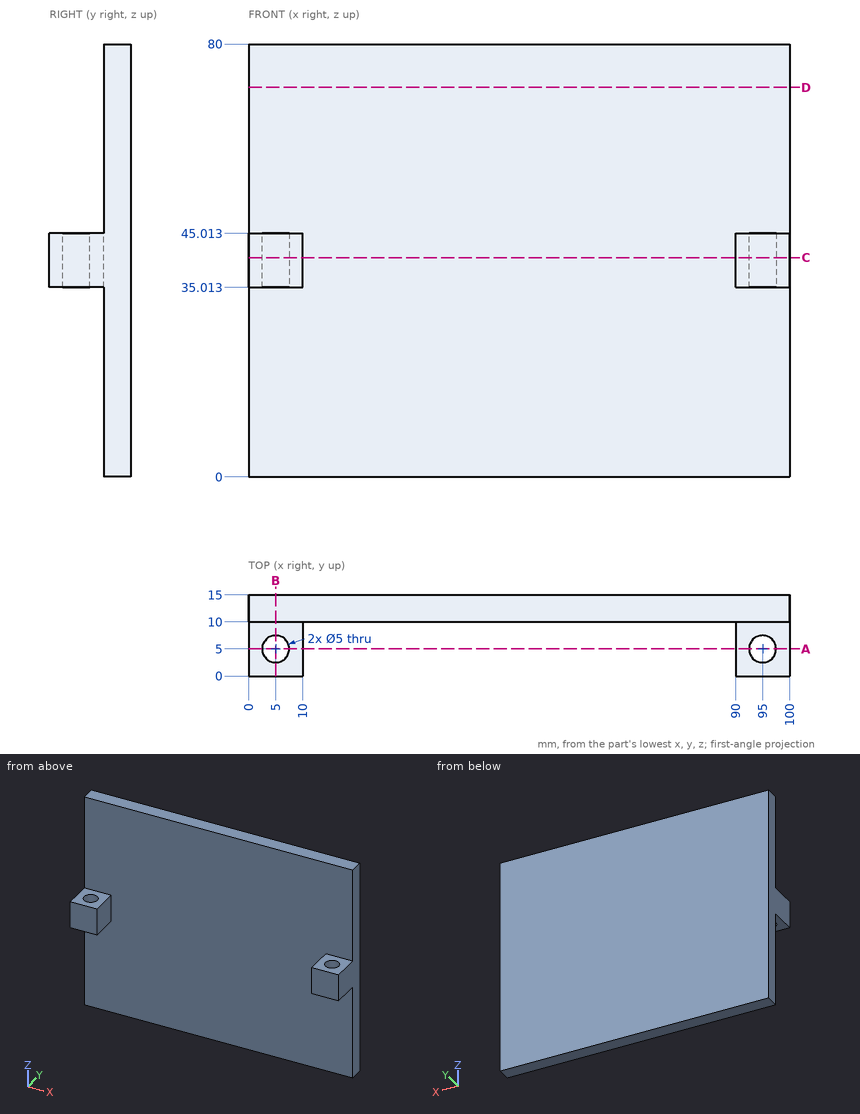
Verification items for this drawing (mm, ordinates from the low corner). Give positions to 0.01 mm unless a question says otherwise; leave off trailing zeros. Loops run counter-clockwise (first coordinate to the right, second up) from the corner with the lowest first, then second, coordinate; pieces in that order, holes last. Notation, with made-up numbers: M 48,-26.75 L 100,-26.75 A8 ccw 100,-19.75 Z; hole C -15.75,-31 d8. An arc over 180 degrees is marked long. Answer as a JSON object with one key per item and string values. Group by question number.
Item 1: Gauge pin test, flat ends, axial feed: pin 1 (3 mm diameter, centred on x = 4, y = 7.5, fed in from +Z); pin 2 (1.5 mm diameter, centred on x = 11.5, y = 5, fed in from +Z); pin 3 (10 mm diameter, centred on x = 79.5, z = 18.5, fed in from -Y); pin 4 (8 mm diameter, centred on x = 97, y = 4.5, fed in from -Z). Record the tip position at first contact, or that the pin passes through.
Item 2: Sectioned sample at D-D on z = 72. Record the boundary of the cut face in (x, y).
Item 3: Sectioned sample at B-B on x = 5. Record the boundary of the cut face in (y, z).
Item 4: Sectioned sample at C-C on z = 40.5. Record the boundary of the cut face in (x, y).
Item 5: Material ranges on L1, parallel to X at y = 2.25, z = 44; L2, parallel to Y at x = 5, z = 38.5; L3, parallel to Y at x = 81, z = 49, recorded low to high.
Item 6: Sectioned sample at A-A on y = 5. Record the boundary of the cut face in (x, z).
Findings below:
{
 "1": {"pin 1": "z = 45.01", "pin 2": "through", "pin 3": "y = 10", "pin 4": "z = 35.01"},
 "2": {"outline": "M 0,10 L 100,10 L 100,15 L 0,15 Z"},
 "3": {"outline": "M 0,35.01 L 2.5,35.01 L 2.5,45.01 L 0,45.01 Z; M 7.5,35.01 L 10,35.01 L 10,0 L 15,0 L 15,80 L 10,80 L 10,45.01 L 7.5,45.01 Z"},
 "4": {"outline": "M 0,0 L 10,0 L 10,10 L 90,10 L 90,0 L 100,0 L 100,15 L 0,15 Z; hole C 5,5 d5; hole C 95,5 d5"},
 "5": {"L1": "0 to 10, 90 to 100", "L2": "0 to 2.5, 7.5 to 15", "L3": "10 to 15"},
 "6": {"outline": "M 0,35.01 L 2.5,35.01 L 2.5,45.01 L 0,45.01 Z; M 7.5,35.01 L 10,35.01 L 10,45.01 L 7.5,45.01 Z; M 90,35.01 L 92.5,35.01 L 92.5,45.01 L 90,45.01 Z; M 97.5,35.01 L 100,35.01 L 100,45.01 L 97.5,45.01 Z"}
}
